Work out the finished part from the listing and answer in its coordinate system (mm). A direction names the side the tool comes from. Round coordinates to 2 decimals unless told otherwise and drop trailing zeros. Write each loop counter-clockwise with the first axis right and the second up, starting at its lowest first coordinate (ties: lowest second). Pieces come first, ordered by that corner, then holes. Notation, with made-up numbers: (83, 47.25) - (136, 47.25) arc R7 cw to (136, 55.25) - close; hole circle Ø10 at (13, 62.25). An arc over 180 degrees is marked (long way). Answer as a JSON object with one key per item and string values.
```python
from build123d import *

# Parameters (mm, degrees)
F1_DEPTH = 14.732
F3_DEPTH = 14.733


with BuildPart() as f1:
    # F0 (on Right) → F1 (new body)
    with BuildSketch(Plane.YZ):
        Polygon((-76.149119, -69.946595), (-76.149119, -76.042595), (-38.049119, -76.042595), (-38.049119, -69.946595), (-47.447119, -69.946595), (-47.447119, -63.342595), (-66.751119, -63.342595), (-66.751119, -69.946595), align=None)
    extrude(amount=F1_DEPTH)

    # F2 (on face) → F3 (cut, through all)
    with BuildSketch(Plane.YZ.offset(14.732)):
        with BuildLine():
            ThreePointArc((-63.703119, -63.342595), (-57.099119, -69.946595), (-50.495119, -63.342595))
            Line((-50.495119, -63.342595), (-63.703119, -63.342595))
        make_face()
    extrude(amount=-F3_DEPTH, mode=Mode.SUBTRACT)


solid = f1.part
```
Item 1: A cutting plane is placed at B-B (x = 3.25). Write down the section's boundary in (y, z).
Results found:
{"outline": "(-76.15, -76.04) - (-38.05, -76.04) - (-38.05, -69.95) - (-47.45, -69.95) - (-47.45, -63.34) - (-50.5, -63.34) arc R6.6 cw to (-63.7, -63.34) - (-66.75, -63.34) - (-66.75, -69.95) - (-76.15, -69.95) - close"}
Item 2: A cutting plane is placed at A-A (z = -67.5). Write down the section's boundary in (x, y).
Results found:
{"outline": "(0, -66.75) - (14.73, -66.75) - (14.73, -62.23) - (0, -62.23) - close; (0, -51.97) - (14.73, -51.97) - (14.73, -47.45) - (0, -47.45) - close"}
Item 3: Determine the mould class of faces 1 (the flat face through (7, -57, -76.043)), 2 (the flat face through (7, -38.049, -73)), 3 (the cylindrical face through (7.469, -57.244, -69.945)), 4 (the flat face through (7, -76.149, -73)) for opening direction Y: pulls with the +Y half, pulls with the -Y half, needs draft (parallel to the pull), parting line crosses it, or undercut.
Results found:
{"face 1": "needs draft", "face 2": "pulls with the +Y half", "face 3": "undercut", "face 4": "pulls with the -Y half"}
Item 4: Each of these flat-tipped pins is pushed along its axis until it touches: P1, Ø5, axis at x = 12.5, z = -66.5, coming from the +Y side; P2, Ø4.5, axis at x = 10, y = -45, coming from the +Z side; P3, Ø5, axis at y = -60.5, z = -65, coming from the -X side. Where does it stop, or does it pass through?
Results found:
{"P1": "y = -47.45", "P2": "z = -69.95", "P3": "through"}
Item 5: A cutting plane is placed at D-D (z = -69). Write down the section's boundary in (x, y), and give its area (3 significant figures).
Results found:
{"outline": "(0, -66.75) - (14.73, -66.75) - (14.73, -60.51) - (0, -60.51) - close; (0, -53.69) - (14.73, -53.69) - (14.73, -47.45) - (0, -47.45) - close", "area": "184 mm²"}
Item 6: Consider line 1 along Y through (x, z) = (7.25, -67.75); line 2 along Y through (x, z) = (9.25, -65.5); line 3 along Z through (x, y) = (2, -74). Determine where each line is inside the solid, lowest interval first.
Results found:
{"line 1": "-66.75 to -62.02, -52.18 to -47.45", "line 2": "-66.75 to -63.34, -50.86 to -47.45", "line 3": "-76.04 to -69.95"}
Item 7: For faces 5 (the flat face through (7, -66.751, -67)), 6 (the flat face through (7, -49, -63.343)), 7 (the flat face through (7, -43, -69.947)), determine the directions among +Z, -Z, +X, -X, +Y, -Y from which every point of the face is accessible in a straight line to the end or side of a thin tool.
Results found:
{"face 5": "+Z, +X, -X, -Y", "face 6": "+Z, +X, -X, +Y, -Y", "face 7": "+Z, +X, -X, +Y"}
Item 8: A cutting plane is placed at C-C (y = -73). Write down the section's boundary in (x, z), and give its area (3 significant figures).
Results found:
{"outline": "(0, -76.04) - (14.73, -76.04) - (14.73, -69.95) - (0, -69.95) - close", "area": "89.8 mm²"}
